Study the drawing (mm; zero at the part's minimum x, y, z) and answer. A direction names the side the tool comes from. Coordinates: 2 decimals unless noted, no trailing zeros. Write each loop counter-clockwise with the first axis right and the second up, starting at its lowest first coordinate (ties: lowest second). Pieces come first, ordered by that corner, then holes. Notation, with made-up numbers: (-16.5, 78) -> (29.5, 78) arc R23 cw to (29.5, 106) -> close; hole circle Ø5 at (-6.5, -7.75). An arc over 180 degrees is marked (long way). Answer in a Markdown table with one row per item. Add a question column.
Item 1: Section D-D on z = 245 is taken. Write down the section's boundary in (x, y).
Item 2: Section A-A on y = 320 is taken. Write down the section's boundary in (x, z), then the cut area to 3 significant figures.
Item 3: Section B-B on x = 320 is taken. Write down the section's boundary in (y, z), then the cut area to 3 significant figures.
Item 4: For a pull along X with two mould halves and no side action, classify the marked faces 1, 2 and 3 as +X half, -X half, draft (parallel to the pull), parting line (faces both ways), or undercut.
Item 5: Given pin 1 Ø6 at (y, z) = (571.5, 339.5) entering from -X; pin 2 Ø3 at (y, z) = (458.5, 41) entering from +X; pin 3 Ø2 at (y, z) = (566.5, 133.5) entering from -X, each flat-ended and moving along its own axis, determine where each tip first touches the part or whether it passes through.
Item 6: Section C-C on z = 101 is taken. Write down the section's boundary in (x, y).
Item 7: Which of the six approach directions +Z, -Z, +X, -X, +Y, -Y give full straight-line access (tool end or side, diameter ignored) to the marked faces 4 and 5?
Item 8: Straight lines are drawn through the part: line 1 (X direction, y = 320, z = 320.5); line 2 (X direction, y = 567, z = 349); line 3 (Y direction, x = 320, z = 244.5). For each, find the intervals that lie inside material, in ascending order. Write a range as from..to.
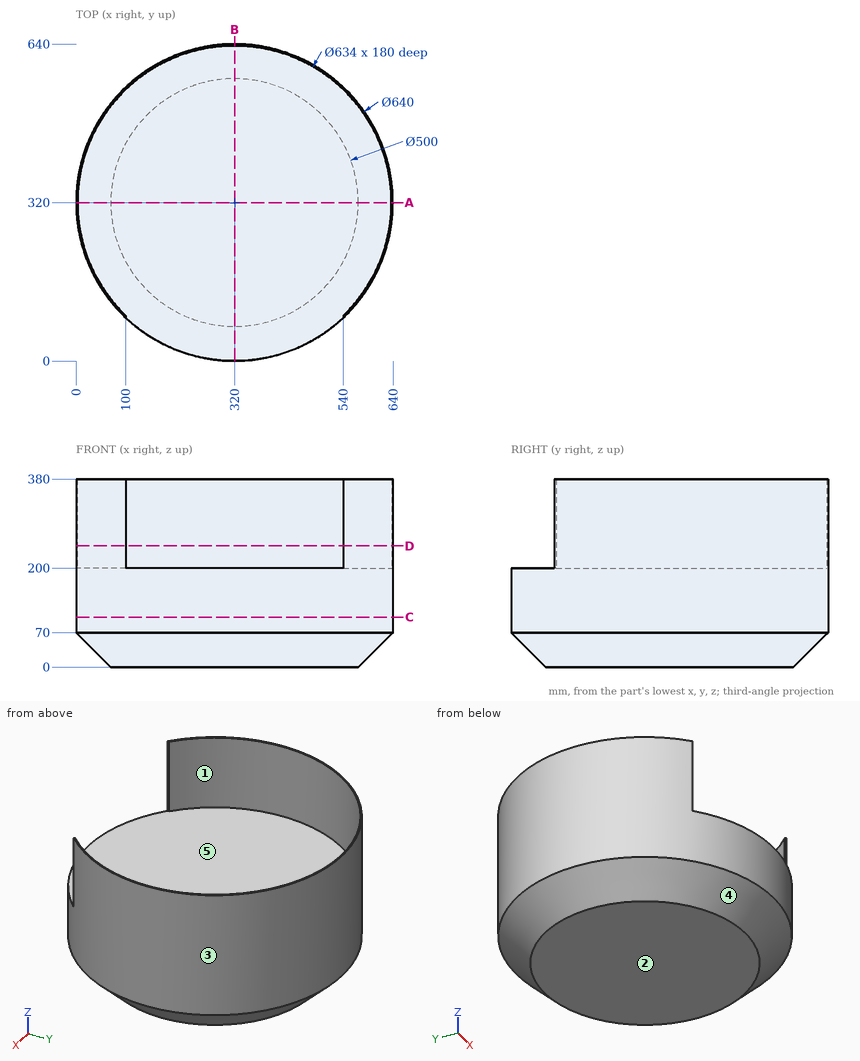
Results below:
| question | item | result |
|---|---|---|
| 1 | outline | (100, 87.62) -> (100, 91.77) arc R317 cw (long way) to (540, 91.77) -> (540, 87.62) arc R320 ccw (long way) to start |
| 2 | outline | (0, 70) -> (70, 0) -> (570, 0) -> (640, 70) -> (640, 380) -> (637, 380) -> (637, 200) -> (3, 200) -> (3, 380) -> (0, 380) -> close |
| 2 | area | 124,000 mm2 |
| 3 | outline | (0, 70) -> (70, 0) -> (570, 0) -> (640, 70) -> (640, 380) -> (637, 380) -> (637, 200) -> (0, 200) -> close |
| 3 | area | 124,000 mm2 |
| 4 | face 1 | undercut |
| 4 | face 2 | draft |
| 4 | face 3 | parting line |
| 5 | pin 1 | stops at x = 118.39 |
| 5 | pin 2 | stops at x = 577.81 |
| 5 | pin 3 | stops at x = 114.74 |
| 6 | outline | circle Ø640 at (320, 320) |
| 7 | face 4 | -Z |
| 7 | face 5 | +Z |
| 8 | line 1 | x = 0..3, 637..640 |
| 8 | line 2 | x = 116.55..121.3, 518.7..523.45 |
| 8 | line 3 | y = 637..640 |
